For this review, take the finished solid that the model builds, in its own axes (mm). Round coordinates to 2 decimals unless told otherwise and drop trailing zeros. Write each loop counter-clockwise with the first axis right and the second up, starting at its lowest first coordinate (ties: lowest second). Pieces come first, ordered by that corner, then holes. Notation, with made-up numbers: (-21.75, 89) -> (-12.75, 89) arc R26 ccw to (-12.75, 109) -> close; hole circle Ø3 at (45.5, 39). An arc over 180 degrees is marked (long way). Write each question's results on one line, items separated by ' | '. Start each with the question number.
Item 1: Add section B-B (z = 5). State the section outline as (x, y) points, plus the area to 3 significant figures.
Item 2: The part is to be moulded in two halves that separate along X. For faces 1 (the cylindrical face through (-7.86, 7.21, 23.06)), 2 (the flat face through (19.05, -3, 4)), 3 (the flat face through (-3, -19.05, 4)), say which applies: +X half, -X half, draft (parallel to the pull), parting line (faces both ways), or undercut.
Item 3: To check wall thickness, follow line 1 along Y through (x, z) = (0, 23); line 2 along X through (y, z) = (10, 6); line 3 along Z through (x, y) = (-1, -15). State the ranges of each line that lie inside material, in increasing order.
Item 4: Add section C-C (x = 6.5). Count the separate pieces of the cut face and the enclosed holes in it, plus the area to 3 significant figures.
from build123d import *

# Parameters (mm, degrees)
F0_W     = 38.1
F0_H     = 38.1
F1_DEPTH = 25.4
F4_DEPTH = 76.2
F6_DEPTH = 76.2
F2_R     = 10.668
F7_DEPTH = 12.7
F8_SIZE  = 5.08


with BuildPart() as f1:
    # F0 (on Top) → F1 (new body)
    with BuildSketch(Plane.XY):
        Rectangle(F0_W, F0_H)
    extrude(amount=F1_DEPTH)

    # F3 (on face) → F4 (cut)
    with BuildSketch(Plane.XZ.offset(19.05)):
        with BuildLine():
            ThreePointArc((0, 21.2725), (-8.5725, 12.7), (0, 4.1275))
            Line((0, 4.1275), (0, 12.7))
            Line((0, 12.7), (0, 21.2725))
        make_face()
        with BuildLine():
            Line((0, 12.7), (0, 4.1275))
            ThreePointArc((0, 4.1275), (6.061673, 6.638327), (8.5725, 12.7))
            ThreePointArc((8.5725, 12.7), (6.061673, 18.761673), (0, 21.2725))
            Line((0, 21.2725), (0, 12.7))
        make_face()
    extrude(amount=-F4_DEPTH, mode=Mode.SUBTRACT)

    # F5 (on face) → F6 (cut)
    with BuildSketch(Plane.YZ.offset(19.05)):
        with BuildLine():
            ThreePointArc((0, 21.2725), (-8.5725, 12.7), (0, 4.1275))
            Line((0, 4.1275), (0, 12.7))
            Line((0, 12.7), (0, 21.2725))
        make_face()
        with BuildLine():
            Line((0, 12.7), (0, 4.1275))
            ThreePointArc((0, 4.1275), (6.061673, 6.638327), (8.5725, 12.7))
            ThreePointArc((8.5725, 12.7), (6.061673, 18.761673), (0, 21.2725))
            Line((0, 21.2725), (0, 12.7))
        make_face()
    extrude(amount=-F6_DEPTH, mode=Mode.SUBTRACT)

    # F2 (on face) → F7 (cut)
    with BuildSketch(Plane.XY.offset(25.4)):
        Circle(F2_R)
    extrude(amount=-F7_DEPTH, mode=Mode.SUBTRACT)

    # F8
    f8_edges = [f1.edges().sort_by_distance(p)[0] for p in [
        (-19.05, 19.05, 12.7),
        (19.05, 19.05, 12.7),
        (19.05, -19.05, 12.7),
        (-19.05, -19.05, 12.7),
    ]]
    chamfer(f8_edges, length=F8_SIZE)


solid = f1.part
Responses:
1) outline: (-19.05, -13.97) -> (-13.97, -19.05) -> (-3.77, -19.05) -> (-3.77, -3.77) -> (-19.05, -3.77) -> close; (-19.05, 3.77) -> (-3.77, 3.77) -> (-3.77, 19.05) -> (-13.97, 19.05) -> (-19.05, 13.97) -> close; (3.77, -19.05) -> (13.97, -19.05) -> (19.05, -13.97) -> (19.05, -3.77) -> (3.77, -3.77) -> close; (3.77, 3.77) -> (19.05, 3.77) -> (19.05, 13.97) -> (13.97, 19.05) -> (3.77, 19.05) -> close | area: 883 mm^2
2) face 1: undercut | face 2: +X half | face 3: draft
3) line 1: y = -19.05 to -10.67, 10.67 to 19.05 | line 2: x = -19.05 to -5.35, 5.35 to 19.05 | line 3: z = 0 to 4.19, 21.21 to 25.4
4) separate pieces: 3 | enclosed holes: 0 | area: 395 mm^2
